from build123d import *

# Parameters (mm, degrees)
SKETCH_1_W      = 11
SKETCH_1_H      = 9.5
EXTRUDE_1_DEPTH = 0.25
SKETCH_2_W      = 11
SKETCH_2_H      = 9.5
SKETCH_2_W_2    = 10.5
SKETCH_2_H_2    = 9.068181818
EXTRUDE_2_DEPTH = 1
EXTRUDE_3_DEPTH = 0.5


with BuildPart() as part:
    # Эскиз1 → Бобышка-Вытянуть1 (new body)
    with BuildSketch(Plane(origin=(0, 0, 0), x_dir=(1, 0, 0), z_dir=(0, 1, 0))):
        Rectangle(SKETCH_1_W, SKETCH_1_H)
    extrude(amount=EXTRUDE_1_DEPTH)

    # Эскиз2 → Бобышка-Вытянуть2 (add)
    with BuildSketch(Plane(origin=(0, 0.25, 0), x_dir=(1, 0, 0), z_dir=(0, 1, 0))):
        Rectangle(SKETCH_2_W, SKETCH_2_H)
        Rectangle(SKETCH_2_W_2, SKETCH_2_H_2, mode=Mode.SUBTRACT)
    extrude(amount=EXTRUDE_2_DEPTH)

    # Эскиз3 → Бобышка-Вытянуть3 (add)
    with BuildSketch(Plane(origin=(0, 0.25, 0), x_dir=(1, 0, 0), z_dir=(0, 1, 0))):
        Polygon((-5.25, 4.534090909), (-4.75, 4.534090909), (-5.25, 4.034090909), align=None)
        Polygon((-5.25, -4.534090909), (-5.25, -4.034090909), (-4.75, -4.534090909), align=None)
        Polygon((5.25, -4.534090909), (5.25, -4.034090909), (4.75, -4.534090909), align=None)
        Polygon((4.75, 4.534090909), (5.25, 4.034090909), (5.25, 4.534090909), align=None)
    extrude(amount=EXTRUDE_3_DEPTH)


solid = part.part
Design review of the part built by this model. Coordinates are the model's own, in mm. A direction names the side the tool comes from. Round coordinates to 2 decimals unless told otherwise and drop trailing zeros. Loops run counter-clockwise (first coordinate to the right, second up) from the corner with the lowest first, then second, coordinate; pieces in that order, holes last. Notation, with made-up numbers: M -30.75,36.5 L -14.75,36.5 A21 ccw -14.75,74.5 Z; hole C 70.25,46.25 d6. An arc over 180 degrees is marked long. Answer as a JSON object with one key per item and string values.
Item 1: Clearance check with a flat-ended pin moving along its axis: P1, Ø2.5, axis at x = 2, z = 0.5, coming from the +Y side. State where the tip first meets the part, or that it passes through.
Answer sheet:
{"P1": "stops at y = 0.25"}
Item 2: We need section C-C on z = 3. Give the boundary of the cut face in (x, y).
Answer sheet:
{"outline": "M -5.5,0 L 5.5,0 L 5.5,1.25 L 5.25,1.25 L 5.25,0.25 L -5.25,0.25 L -5.25,1.25 L -5.5,1.25 Z"}
Item 3: Machinability: for faces 5 (the flat face through (5.25, 1, 0)), 6 (the flat face through (0, 1, 4.75)), which of the approach directions +Z, -Z, +X, -X, +Y, -Y give a long, thin tool a straight path to every point of the face, cutting with its end or side? Answer none if there is none.
Answer sheet:
{"face 5": "+Y", "face 6": "+Z, +X, -X, +Y, -Y"}
Item 4: We need section B-B on x = -3.5. Give the boundary of the cut face in (y, z), and give its area (3 significant figures).
Answer sheet:
{"outline": "M 0,-4.75 L 1.25,-4.75 L 1.25,-4.53 L 0.25,-4.53 L 0.25,4.53 L 1.25,4.53 L 1.25,4.75 L 0,4.75 Z", "area": "2.81 mm^2"}
Item 5: The part is to be moulded in two halves that separate along X. For faces 1 (the flat face through (0, 1, -4.75)), 2 (the flat face through (-5.5, 1, 0)), 3 (the flat face through (0, 1, -4.534)), 4 (the flat face through (5.5, 1, 0)), say which applies: pulls with the +X half, pulls with the -X half, needs draft (parallel to the pull), parting line crosses it, or undercut.
Answer sheet:
{"face 1": "needs draft", "face 2": "pulls with the -X half", "face 3": "undercut", "face 4": "pulls with the +X half"}
Item 6: We need section A-A on y = 0.9. Give the boundary of the cut face in (x, z), and give its area (3 significant figures).
Answer sheet:
{"outline": "M -5.5,-4.75 L 5.5,-4.75 L 5.5,4.75 L -5.5,4.75 Z; hole M -5.25,-4.53 L 5.25,-4.53 L 5.25,4.53 L -5.25,4.53 Z", "area": "9.28 mm^2"}
Item 7: Wall thickness on L1, parallel to X at y = 0.65, z = -3.75; L2, parallel to Z at x = 3, y = 0.95; L3, parallel to Y at x = 3.5, z = 2: over which ranges is each line inside the solid? List them lowest first. Write a range as from..to.
Answer sheet:
{"L1": "x = -5.5..-5.25, 5.25..5.5", "L2": "z = -4.75..-4.53, 4.53..4.75", "L3": "y = 0..0.25"}
